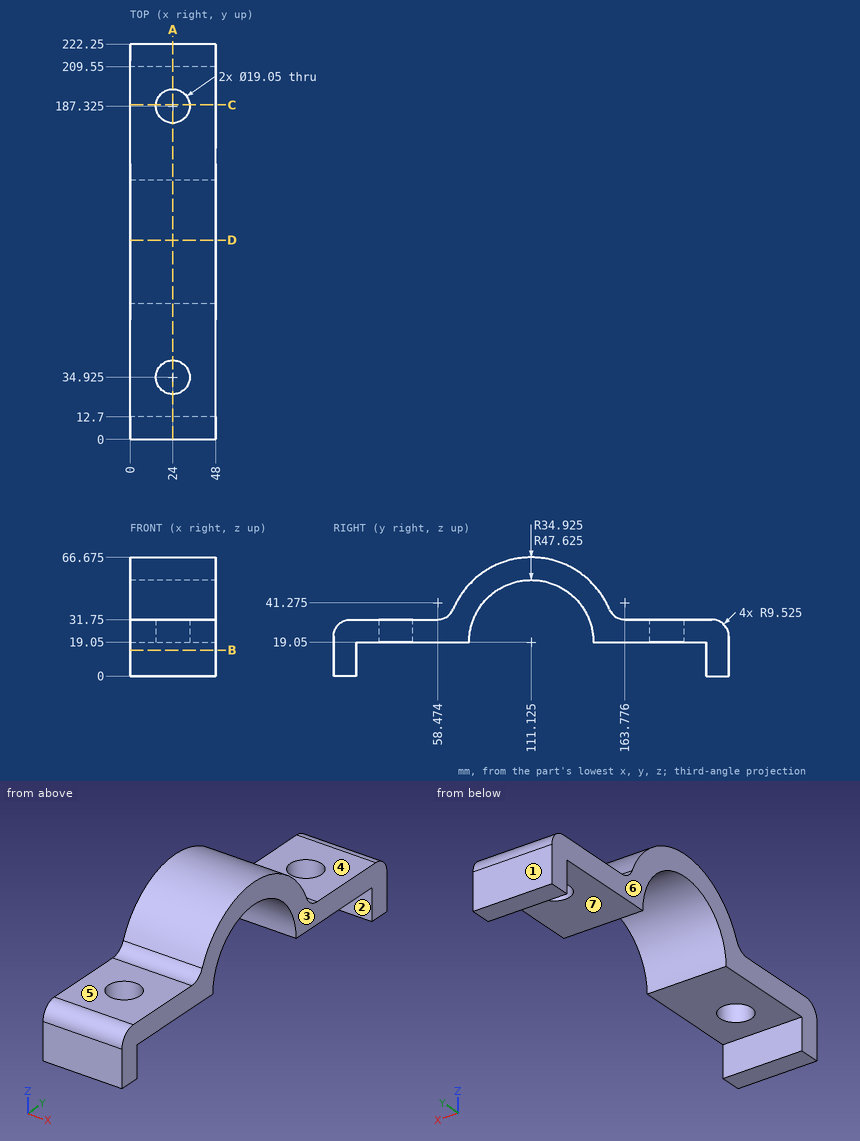
Verification items for this drawing (mm, ordinates from the low corner). A direction names the side the tool comes from. Give positions to 0.01 mm unless a question says otherwise; leave off trailing zeros. Write each loop counter-clockwise with the first axis right and the second up, starting at its lowest first coordinate (ties: lowest second). Pieces come first, ordered by that corner, then holes.
1) Material ranges on L1, parallel to Y at x = 3, z = 20.5; L2, parallel to Y at x = 20, z = 26; L3, parallel to Z at x = 38, y = 35.5, recorded low to high.
2) Section check D-D, the plane y = 112. Record the boundary of the cut face in (x, z), and give its area (3 significant figures).
3) Gauge pin test, flat ends, axial feed: pin 1 (9.5 mm diameter, centred on x = 23.5, z = 6, fed in from -Y); pin 2 (12 mm diameter, centred on x = 36, y = 127, fed in from -Z) (1 decimal); pin 3 (3 mm diameter, centred on x = 8, z = 32.5, fed in from +Y); pin 4 (24 mm diameter, centred on x = 30, y = 179, fed in from +Z). Record the tip position at first contact, or that the pin passes through.
4) Section check B-B, the plane z = 14.5. Record the boundary of the cut face in (x, y), and give its area (3 significant figures).
5) Release check for a two-part mould opening along Y. For the marked faces 1, 2 and 3 record: pulls with the +Y half, pulls with the -Y half, needs draft (parallel to the pull), parting line crosses it, or undercut.
6) Section check C-C, the plane y = 188. Record the boundary of the cut face in (x, z), and give its area (3 significant figures).
7) Access from +Z, -Z, +X, -X, +Y, -Y to the whole of each face (thin tool, end or side, straight path). Record for the marked faces 4, 5, 6 and 7.
8) Section check A-A, the plane x = 24. State how many separate pieces and enclosed holes the cut face has, and give its area (3 significant figures).
Computed:
1. L1: y = 0 to 76.23, 146.02 to 222.25
1. L2: y = 0.78 to 26.28, 43.57 to 76.9, 145.35 to 178.68, 195.97 to 221.47
1. L3: z = 19.05 to 31.75
2. outline: (0, 53.96) - (48, 53.96) - (48, 66.67) - (0, 66.67) - close
2. area: 610 mm2
3. pin 1: stops at y = 0
3. pin 2: stops at z = 46.3
3. pin 3: stops at y = 216.43
3. pin 4: stops at z = 31.75
4. outline: (0, 0) - (48, 0) - (48, 12.7) - (0, 12.7) - close; (0, 209.55) - (48, 209.55) - (48, 222.25) - (0, 222.25) - close
4. area: 1,220 mm2
5. face 1: pulls with the +Y half
5. face 2: undercut
5. face 3: needs draft
6. outline: (0, 19.05) - (14.5, 19.05) - (14.5, 31.75) - (0, 31.75) - close; (33.5, 19.05) - (48, 19.05) - (48, 31.75) - (33.5, 31.75) - close
6. area: 368 mm2
7. face 4: +Z, +X, -X, +Y
7. face 5: +Z, +X, -X, -Y
7. face 6: +Z, -Z, -X, +Y, -Y
7. face 7: -Z, +X, -X
8. separate pieces: 3
8. enclosed holes: 0
8. area: 3,250 mm2
